Can you work these out from the model? Positions are in its coordinate system, mm. Give positions to 0.01 mm unless a question says otherwise; leave off trailing zeros. Order: outer loops, then holes, each group sorted by start corner. A loop starts at its lowest first (then second) coordinate and runs counter-clockwise, first axis right, second up. Notation, with made-up numbers: (8.5, 13) - (43.5, 13) arc R30 cw to (43.5, 43) - close; hole circle Ø1 at (80.5, 63). An arc over 180 degrees is marked (long way). Answer as CSV lines item,"result".
```python
from build123d import *

# Parameters (mm, degrees)
SKETCH1_R           = 1.445304889
BOSS_EXTRUDE1_DEPTH = 3
SKETCH2_R           = 0.75
CUT_EXTRUDE1_DEPTH  = 10
SKETCH3_R           = 0.657732985
CUT_EXTRUDE2_DEPTH  = 4
SKETCH4_R           = 0.657732985
CUT_EXTRUDE3_DEPTH  = 4


with BuildPart() as part:
    # Sketch1 → Boss-Extrude1 (new body)
    with BuildSketch(Plane.XY):
        with BuildLine():
            Line((2.709665951, -9.119248637), (4.330233257, 6.26308765))
            ThreePointArc((4.330233257, 6.26308765), (3.57642555, 8.584523689), (1.346744655, 9.577405579))
            ThreePointArc((1.346744655, 9.577405579), (-0.88293624, 8.584523689), (-1.636743947, 6.26308765))
            Line((-1.636743947, 6.26308765), (-0.016176641, -9.119248637))
            Line((-0.016176641, -9.119248637), (0.013745769, -9.403270519))
            ThreePointArc((0.013745769, -9.403270519), (1.346744655, -10.482169933), (2.679743541, -9.403270519))
            Line((2.679743541, -9.403270519), (2.709665951, -9.119248637))
        make_face()
        with Locations((1.346744655, 6.577405579)):
            Circle(SKETCH1_R, mode=Mode.SUBTRACT)
    extrude(amount=BOSS_EXTRUDE1_DEPTH)

    # Sketch2 → Cut-Extrude1 (cut)
    with BuildSketch(Plane.XY.offset(3)):
        with Locations((1.346744655, -8.903103928)):
            Circle(SKETCH2_R)
    extrude(amount=-CUT_EXTRUDE1_DEPTH, mode=Mode.SUBTRACT)

    # Sketch3 → Cut-Extrude2 (cut, through all)
    with BuildSketch(Plane(origin=(0, 0, 0), x_dir=(-1, 0, 0), z_dir=(0, 0, -1))):
        with Locations((-1.275359723, -0.820045285)):
            Circle(SKETCH3_R)
    extrude(amount=-CUT_EXTRUDE2_DEPTH, mode=Mode.SUBTRACT)

    # Sketch4 → Cut-Extrude3 (cut, through all)
    with BuildSketch(Plane(origin=(0, 0, 0), x_dir=(-1, 0, 0), z_dir=(0, 0, -1))):
        with Locations((-1.43062658, -4.837170951)):
            Circle(SKETCH4_R)
    extrude(amount=-CUT_EXTRUDE3_DEPTH, mode=Mode.SUBTRACT)


solid = part.part
```
1) I want a section at A-A on y = 6.75. Write out the boundary of the cut face in (x, z).
Answer block:
outline,"(-1.65, 0) - (-0.09, 0) - (-0.09, 3) - (-1.65, 3) - close; (2.78, 0) - (4.34, 0) - (4.34, 3) - (2.78, 3) - close"
2) I'm going to push a flat-ended pin straight in: P1, Ø1, axis at y = 7, z = 1, coming from the +X side. Where does the tip first touch, or does it pass through?
Answer block:
P1,"x = 4.35"
3) I want a section at C-C on z = 2.65. Write out the boundary of the cut face in (x, y), plus the area to 3 significant figures.
Answer block:
outline,"(-1.64, 6.26) - (0.01, -9.4) arc R1.36 ccw to (2.68, -9.4) - (4.33, 6.26) arc R3 ccw (long way) to start; hole circle Ø2.89 at (1.35, 6.58); hole circle Ø1.5 at (1.35, -8.9); hole circle Ø1.32 at (1.28, -0.82); hole circle Ø1.32 at (1.43, -4.84)"
area,"74.7 mm2"
4) I need wall thicknesses on line 1 along X through (y, z) = (6.5, 0.25); line 2 along Y through (x, z) = (1.4, 0.9) (3 decimals); line 3 along Y through (x, z) = (1.5, 2.75). Which ranges of each line are inside material? Lowest first, please. Write a range as [from, to].
Answer block:
line 1,"[-1.65, -0.1], [2.79, 4.35]"
line 2,"[-10.481, -9.651], [-8.155, -5.494], [-4.18, -1.466], [-0.174, 5.133], [8.022, 9.577]"
line 3,"[-10.47, -9.64], [-8.17, -5.49], [-4.18, -1.44], [-0.2, 5.14], [8.01, 9.57]"
5) I want a section at B-B on x = 1.05. Write out the boundary of the cut face in (y, z), plus the area to 3 significant figures.
Answer block:
outline,"(-10.45, 0) - (-9.59, 0) - (-9.59, 3) - (-10.45, 3) - close; (-8.21, 0) - (-5.37, 0) - (-5.37, 3) - (-8.21, 3) - close; (-4.3, 0) - (-1.44, 0) - (-1.44, 3) - (-4.3, 3) - close; (-0.2, 0) - (5.16, 0) - (5.16, 3) - (-0.2, 3) - close; (7.99, 0) - (9.56, 0) - (9.56, 3) - (7.99, 3) - close"
area,"40.5 mm2"
6) I want a section at D-D on y = 2. Write out the boundary of the cut face in (x, z).
Answer block:
outline,"(-1.19, 0) - (3.88, 0) - (3.88, 3) - (-1.19, 3) - close"
7) If we mould it in two halves opening along Y, with no side actions, what happens to faces 1 (the cylindrical face through (1.32, -10.48, 1.48)), 2 (the flat face through (1, 2, 0)), 3 (the cylindrical face through (1.76, -0.376, 1.479))? For each: +Y half, -Y half, draft (parallel to the pull), parting line (faces both ways), or undercut.
Answer block:
face 1,"-Y half"
face 2,"draft"
face 3,"undercut"
